```python
from build123d import *

# Parameters (mm, degrees)
F0_W        = 51.0822050273
F0_H        = 117.4111329019
F1_DEPTH    = 25.4
F2_DEPTH    = 76.7365470529
F3_W        = 51.0822050273
F3_H        = 53.3235035837
F4_DEPTH    = 61.1563976854
F5_T1_DEPTH = 365.1602492866


# Not quite as in the source:
# - a fillet or chamfer that OpenCascade refuses, or shapes differently, is made with other operations: its cross-section is extruded or revolved along the edge and cut away or added


with BuildPart() as f1:
    # F0 (on Front) → F1 (new body)
    with BuildSketch(Plane.XZ):
        with Locations((-25.5411025137, 1.6260724515)):
            Rectangle(F0_W, F0_H)
    extrude(amount=F1_DEPTH)

    # F2 (add): a face of the model
    f2_faces = [f1.faces().sort_by_distance(p)[0] for p in [
        (-25.5411025137, -12.7, 60.3316389024),
    ]]
    extrude(f2_faces, amount=F2_DEPTH)

    # F3 (on face) → F4 (join)
    with BuildSketch(Plane.XZ.offset(25.4)):
        with Locations((-25.5411025137, 110.4064341635)):
            Rectangle(F3_W, F3_H)
    extrude(amount=F4_DEPTH)

    # F5: chamfer of 60.96 x 53.34 on 1 edges, made by hand

    # F5_s2 → F5_t1 (cut)
    with BuildSketch(Plane.YZ.offset(-208.121227157)):
        Polygon((-25.5963976854, 83.7446823716), (-86.5563976854, 137.0846823716), (-86.5563976854, 83.7446823716), align=None)
    extrude(amount=F5_T1_DEPTH, mode=Mode.SUBTRACT)


solid = f1.part
```
CAD build for the part. Positions are in the model's coordinates, mm. A direction names the side the tool comes from. Coordinates: 2 decimals unless noted, no trailing zeros. Write each loop counter-clockwise with the first axis right and the second up, starting at its lowest first coordinate (ties: lowest second). Pieces come first, ordered by that corner, then holes.
(1) Cut at B-B, the plane z = -34. List the corners of the cut face in (x, y), and give its area (3 significant figures).
(2) 3-axis set-ups, long thin cutter, end or side, ignore diameter. For faces 1 (the face through (-26, -25.4, 12)), 2 (the face through (-26, -13, -57.079)): which of +Z, -Z, +X, -X, +Y, -Y reach the whole face in a straight line?
(3) Drill centre lines: probe 1 along Y at (x, z) = (-16.5, 47.5); probe 2 along Y at (x, z) = (-23.5, 85.5); probe 3 along Z at (x, y) = (-30, -25.5). Where is each one in solid material? Low to high.
(4) Cut at C-C, the plane y = -29. List the corners of the cut face in (x, z), and give its area (3 significant figures).
(5) Flat gauge pins, fed straight in: pin 1 (1 mm diameter, centred on x = -38.5, z = 34, fed in from -Y); pin 2 (12 mm diameter, centred on x = -40.5, y = -45.5, fed in from -Z); pin 3 (2 mm diameter, centred on x = -31.5, y = -68.5, fed in from -Z). Where does each tip first touch, or does it go through?
(6) Cut at A-A, the plane x = -34. List the corners of the cut face in (y, z), and give its area (3 significant figures).
Geometry says:
1. outline: (-51.08, -25.4) - (0, -25.4) - (0, 0) - (-51.08, 0) - close
1. area: 1,300 mm2
2. face 1: -Z, +X, -X, -Y
2. face 2: -Z, +X, -X, +Y, -Y
3. probe 1: y = -25.4 to 0
3. probe 2: y = -27.6 to 0
3. probe 3: z = 83.74 to 137.07
4. outline: (-51.08, 86.72) - (0, 86.72) - (0, 137.07) - (-51.08, 137.07) - close
4. area: 2,570 mm2
5. pin 1: stops at y = -25.4
5. pin 2: stops at z = 95.91
5. pin 3: stops at z = 120.41
6. outline: (-86.54, 137.07) - (-25.6, 83.74) - (-25.4, 83.74) - (-25.4, -57.08) - (0, -57.08) - (0, 137.07) - close
6. area: 6,570 mm2
